Here's how the part is built. I have some questions about the finished solid (model axes, mm). Coordinates: 2 decimals unless noted, no trailing zeros. Loops run counter-clockwise (first coordinate to the right, second up) from the corner with the lowest first, then second, coordinate; pieces in that order, holes last.
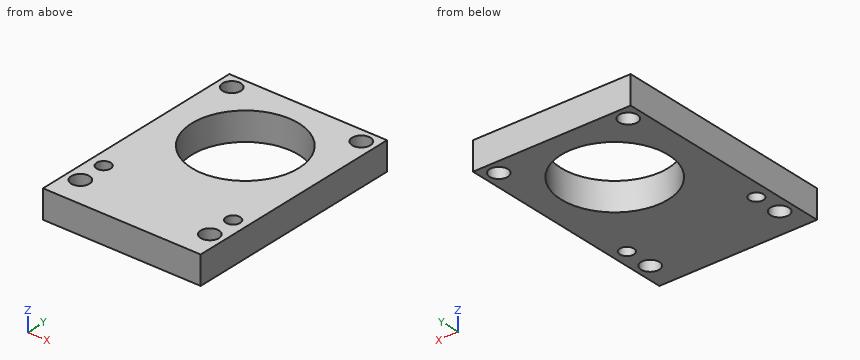
from build123d import *

# Parameters (mm, degrees)
F0_W     = 56
F0_H     = 80
F1_DEPTH = 10
F2_R     = 19
F3_DEPTH = 10.001
F4_R     = 3.25
F5_DEPTH = 10.001
F6_R     = 2.5
F7_DEPTH = 10.001


with BuildPart() as f1:
    # F0 (on Top) → F1 (new body)
    with BuildSketch(Plane.XY):
        with Locations((0, -13)):
            Rectangle(F0_W, F0_H)
    extrude(amount=F1_DEPTH)

    # F2 (on face) → F3 (cut, through all)
    with BuildSketch(Plane.XY.offset(10)):
        Circle(F2_R)
    extrude(amount=-F3_DEPTH, mode=Mode.SUBTRACT)

    # F4 (on face) → F5 (cut, through all)
    with BuildSketch(Plane.XY.offset(10)):
        with Locations((-23, 22)):
            Circle(F4_R)
        with Locations((-23, -43)):
            Circle(F4_R)
        with Locations((23, 22)):
            Circle(F4_R)
        with Locations((23, -43)):
            Circle(F4_R)
    extrude(amount=-F5_DEPTH, mode=Mode.SUBTRACT)

    # F6 (on face) → F7 (cut, through all)
    with BuildSketch(Plane.XY.offset(10)):
        with Locations((-23, -33)):
            Circle(F6_R)
        with Locations((23, -33)):
            Circle(F6_R)
    extrude(amount=-F7_DEPTH, mode=Mode.SUBTRACT)


solid = f1.part
Q1. Please list where these lines run through material, in increasing order: probe 1 along Y at (x, z) = (23, 2.75); probe 2 along Y at (x, z) = (-22, 3.75); probe 3 along X at (y, z) = (-42, 9).
Q2. Suppose I cut it at D-D on x = 0. Write out the boundary of the cut face in (y, z), and give its area (3 significant figures).
Q3. Suppose I cut it at B-B on y = -43. Write out the boundary of the cut face in (x, z), and give its area (3 significant figures).
Q4. Suppose I cut it at C-C on z = 6.75. Write out the boundary of the cut face in (x, y).
Q5. Suppose I cut it at A-A on x = 23. Write out the boundary of the cut face in (y, z), and give its area (3 significant figures).
Check values:
1. probe 1: y = -53 to -46.25, -39.75 to -35.5, -30.5 to 18.75, 25.25 to 27
1. probe 2: y = -53 to -46.09, -39.91 to -35.29, -30.71 to 18.91, 25.09 to 27
1. probe 3: x = -28 to -26.09, -19.91 to 19.91, 26.09 to 28
2. outline: (-53, 0) - (-19, 0) - (-19, 10) - (-53, 10) - close; (19, 0) - (27, 0) - (27, 10) - (19, 10) - close
2. area: 420 mm2
3. outline: (-28, 0) - (-26.25, 0) - (-26.25, 10) - (-28, 10) - close; (-19.75, 0) - (19.75, 0) - (19.75, 10) - (-19.75, 10) - close; (26.25, 0) - (28, 0) - (28, 10) - (26.25, 10) - close
3. area: 430 mm2
4. outline: (-28, -53) - (28, -53) - (28, 27) - (-28, 27) - close; hole circle Ø6.5 at (-23, -43); hole circle Ø6.5 at (-23, 22); hole circle Ø5 at (-23, -33); hole circle Ø38 at (0, 0); hole circle Ø6.5 at (23, -43); hole circle Ø6.5 at (23, 22); hole circle Ø5 at (23, -33)
5. outline: (-53, 0) - (-46.25, 0) - (-46.25, 10) - (-53, 10) - close; (-39.75, 0) - (-35.5, 0) - (-35.5, 10) - (-39.75, 10) - close; (-30.5, 0) - (18.75, 0) - (18.75, 10) - (-30.5, 10) - close; (25.25, 0) - (27, 0) - (27, 10) - (25.25, 10) - close
5. area: 620 mm2
